```python
from build123d import *

# Parameters (mm, degrees)
EXTRUDE_1_DEPTH     = 10
SKETCH_2_W          = 30
SKETCH_2_H          = 10
EXTRUDE_2_DEPTH     = 267.5
SKETCH_3_W          = 25
SKETCH_3_H          = 309.1
CUT_EXTRUDE_1_DEPTH = 5
CUT_EXTRUDE_1_DRAFT = -25
CUT_EXTRUDE_2_DEPTH = 296.795216324
SKETCH_5_R          = 1.25
CUT_EXTRUDE_3_DEPTH = 10
SKETCH_6_W          = 20.368461709
SKETCH_6_H          = 6.660502167
CUT_EXTRUDE_4_DEPTH = 400


with BuildPart() as part:
    # 스케치1 → 보스-돌출1 (new body)
    with BuildSketch(Plane.XY):
        Polygon((0, 0), (-30, 0), (-30, 2.5), (-17.95, 14.55), (-12.05, 14.55), (0, 2.5), align=None)
    extrude_1 = extrude(amount=EXTRUDE_1_DEPTH)

    # 스케치2 → 보스-돌출2 (add)
    with BuildSketch(Plane.XZ):
        with Locations((-15, 5)):
            Rectangle(SKETCH_2_W, SKETCH_2_H)
    extrude(amount=EXTRUDE_2_DEPTH)

    # 대칭 복사1: 보스-돌출1 across plane
    add(extrude_1.mirror(Plane(origin=(0, -132.5, 0), x_dir=(0, 0, 1), z_dir=(0, -1, 0))))


with BuildPart() as cut_extrude_1_tool:
    # 스케치3 → 컷-돌출1 (with draft: the straight prism first)
    with BuildSketch(Plane.XY.offset(10)):
        with Locations((-15, -140)):
            Rectangle(SKETCH_3_W, SKETCH_3_H)
    extrude(amount=-CUT_EXTRUDE_1_DEPTH)
    # 컷-돌출1: the draft: its side faces are tilted about the plane it starts from
    cut_extrude_1_sides = [cut_extrude_1_tool.faces().sort_by_distance(p)[0] for p in [
        (-27.5, -140, 7.5),
        (-15, -294.55, 7.5),
        (-2.5, -140, 7.5),
        (-15, 14.55, 7.5),
    ]]
    draft(cut_extrude_1_sides, Plane.XY.offset(10), CUT_EXTRUDE_1_DRAFT)


with BuildPart() as part_1:
    add(part.part)

    # 컷-돌출1: cut by cut_extrude_1_tool
    add(cut_extrude_1_tool.part, mode=Mode.SUBTRACT)

    # 스케치4 → 컷-돌출2 (cut, through all)
    with BuildSketch(Plane.XZ.offset(279.55)):
        Polygon((-27.5, 10), (-2.5, 10), (-14.35, 5), (-25.2, 5), align=None)
    extrude(amount=-CUT_EXTRUDE_2_DEPTH, mode=Mode.SUBTRACT)

    # 스케치5 → 컷-돌출3 (cut)
    with BuildSketch(Plane.XY.offset(10)):
        with Locations((-10, 2.55)):
            Circle(SKETCH_5_R)
        with Locations((-20, 2.55)):
            Circle(SKETCH_5_R)
    cut_extrude_3 = extrude(amount=-CUT_EXTRUDE_3_DEPTH, mode=Mode.SUBTRACT)

    # 대칭 복사2: 컷-돌출3 across plane
    add(cut_extrude_3.mirror(Plane(origin=(0, -132.5, 0), x_dir=(0, 0, 1), z_dir=(0, -1, 0))), mode=Mode.SUBTRACT)

    # 스케치6 → 컷-돌출4 (cut)
    with BuildSketch(Plane.XZ.offset(279.55)):
        with Locations((-15.015769146, 8.330251084)):
            Rectangle(SKETCH_6_W, SKETCH_6_H)
    extrude(amount=-CUT_EXTRUDE_4_DEPTH, mode=Mode.SUBTRACT)


solid = part_1.part
```
Source: CAD feature listing. Evaluate the final solid. Frame: model axes, mm. A direction names the side the tool comes from. Give positions to 0.01 mm unless a question says otherwise; leave off trailing zeros. Loops run counter-clockwise (first coordinate to the right, second up) from the corner with the lowest first, then second, coordinate; pieces in that order, holes last. Notation, with made-up numbers: (-23.5, 84.25) -> (33.5, 84.25) arc R9 cw to (33.5, 99.25) -> close; hole circle Ø7 at (86.5, -16.75). An arc over 180 degrees is marked (long way). Put each result on its own line as item: value. Start each with the question number.
1) Reachability of faces 5 (the face through (-15, -279.55, 2)), 6 (the face through (-15, -130, 5)) from +Z, -Z, +X, -X, +Y, -Y: full face, straight path, thin tool, end or side. Return the list, or none.
2) Draft query along X for faces 1 (the face through (-3.65, -134.46, 7.53)), 2 (the face through (-26.33, -134.46, 7.46)), 3 (the face through (-4.8, 7.3, 3.8)), 4 (the face through (-15, 14.55, 2)). Return one class per face: released by +X, released by -X, zero draft, split by the parting line, or undercut.
3) Cut plane A-A (y = -4.5). Return loops of the section in (x, z), then the cut area to 3 significant figures.
4) Contact query for flat-ended pins moving along their axis: P1, Ø6, axis at x = -18, y = -124.5, coming from the +Z side; P2, Ø3, axis at x = -24, z = 6, coming from the +Y side; P3, Ø2, axis at x = -5, z = 5, coming from the -Y side. Output: stop coordinate, or through.
5) Material intervals for probe 1 along Y at (x, z) = (-20, 3.7); probe 2 along X at (y, z) = (1.5, 3.5); probe 3 along Z at (x, y) = (-16.25, -228.5), sorted ascending.
6) Cut plane B-B (z = 7.25). Return loops of the section in (x, y) (3 decimals).
Results are:
1. face 5: +Z, -Z, +X, -X, -Y
1. face 6: +Z, +Y, -Y
2. face 1: undercut
2. face 2: undercut
2. face 3: released by +X
2. face 4: zero draft
3. outline: (-30, 0) -> (0, 0) -> (0, 10) -> (-2.5, 10) -> (-4.83, 5) -> (-25.2, 5) -> (-27.5, 10) -> (-30, 10) -> close
3. area: 187 mm2
4. P1: stops at z = 5
4. P2: stops at y = 9.62
4. P3: stops at y = -273.5
5. probe 1: y = -277.5 to -268.8, -266.3 to 1.3, 3.8 to 12.5
5. probe 2: x = -30 to -20.68, -19.32 to -10.68, -9.32 to 0
5. probe 3: z = 0 to 5
6. outline: (-30, -267.5) -> (-26.235, -271.265) -> (-26.235, 6.265) -> (-30, 2.5) -> close; (-3.782, -271.282) -> (0, -267.5) -> (0, 2.5) -> (-3.782, 6.282) -> close
